```python
from build123d import *

# Parameters (mm, degrees)
CONG_0_2_R = 0.2
CONG_1_2_R = 1.2


with BuildPart() as part:
    # Esquisse1 → Base-Révolution (revolve)
    with BuildSketch(Plane(origin=(0, -0.000542726, 1021.101133201), x_dir=(1, 0, 0), z_dir=(0, -5.315106892389565e-07, 0.9999999999998588))):
        Polygon((1715.401443519, 541.998878787), (1711.40144353, 541.999169346), (1711.400935051, 534.999169365), (1712.400935049, 534.999096725), (1712.401370888, 540.999096709), (1715.40137088, 540.99887879), align=None)
    revolve(axis=Axis((1705.401443602, 541.999832964, 1021.10142128), (-7.263980373159368e-05, -0.9999999973615882, -5.315107006836232e-07)))

    # Congé0.2
    cong_0_2_edges = [part.edges().sort_by_distance(p)[0] for p in [
        (1698.401370924, 540.99957094, 1021.101420749),
    ]]
    fillet(cong_0_2_edges, radius=CONG_0_2_R)

    # Congé1.2
    cong_1_2_edges = [part.edges().sort_by_distance(p)[0] for p in [
        (1699.401443562, 541.999498298, 1021.10142128),
    ]]
    fillet(cong_1_2_edges, radius=CONG_1_2_R)


solid = part.part
```
Could you check a few things on this model? Use its own coordinates, in mm. Give positions to 0.01 mm unless a question says otherwise; leave off trailing zeros.
Q1. We'd pull the mould along Z, two halves only. Please class faces 1 (the cylindrical face through (1711.124, 537.858, 1022.904)), 2 (the cylindrical face through (1695.41, 541.51, 1021.54)): +Z half, -Z half, draft (parallel to the pull), parting line (faces both ways), or undercut.
Q2. If I drill on line 1 along X through (y, z) = (536.5, 1024.5); line 2 along X through (y, z) = (540.75, 1024); line 3 along Y through (x, z) = (1714, 1016.5), over which ranges is the centre line in solid material (lowest first)?
Q3. I'm going to push flat-ended pins straight in: P1, Ø1, axis at x = 1706.5, z = 1015.5, coming from the +Y side; P2, Ø3, axis at x = 1710.5, z = 1015, coming from the -Y side; P3, Ø1.5, axis at x = 1713, z = 1015.5, coming from the -Y side; P4, Ø1, axis at x = 1707, y = 540, coming from the -Z side. Where does each tip first touch, or does it pass through?
Solution:
1. face 1: undercut
1. face 2: parting line
2. line 1: x = 1699.28 to 1700.46, 1710.35 to 1711.52
2. line 2: x = 1699.03 to 1700.15, 1710.65 to 1711.77
2. line 3: y = 541 to 542
3. P1: stops at y = 541.47
3. P2: stops at y = 535
3. P3: stops at y = 541
3. P4: stops at z = 1014.19
